Could you check a few things on this drawing? It's one solid part, dimensions in mm from its lowest x, y, z. A direction names the side the tool comes from. Give positions to 0.01 mm unless a question says otherwise; leave off trailing zeros. Write each loop counter-clockwise with the first axis right and the second up, starting at its lowest first coordinate (ties: lowest second). Pieces come first, ordered by that corner, then holes. Notation, with made-up numbers: (31.5, 23) - (69.5, 23) arc R14 cw to (69.5, 29) - close; hole circle Ø9 at (29.25, -17). An arc over 180 degrees is marked (long way). One line per item, written item: value. Start each with the question number.
1) On a 3-axis mill with a long thin cutter (end or side, diameter ignored), from which of +Z, -Z, +X, -X, +Y, -Y can I reach the whole of each face in a straight line? I mean the marked faces 1, 2 and 3. Say none if no direction works.
2) Imagine slicing it at B-B on x = 4. Write out the boundary of the cut face in (y, z).
3) Imagine slicing it at C-C on y = 8. Write out the boundary of the cut face in (x, z), plus the area to 3 significant figures.
4) Imagine slicing it at A-A on z = 4. Write out the boundary of the cut face in (x, y).
5) Please list where these lines run through material, in increasing order: L1, parallel to Y at x = 6.5, z = 3.75; L2, parallel to X at y = 7, z = 4; L3, parallel to X at y = 44.5, z = 1.5. Write a range as [from, to].
6) Imagine slicing it at D-D on y = 25.5. Write out the boundary of the cut face in (x, z).
7) I'm going to push a flat-ended pin straight in: P1, Ø1.5, axis at y = 11.5, z = 6.5, coming from the +X side. Where does the tip first touch, or does it pass through?
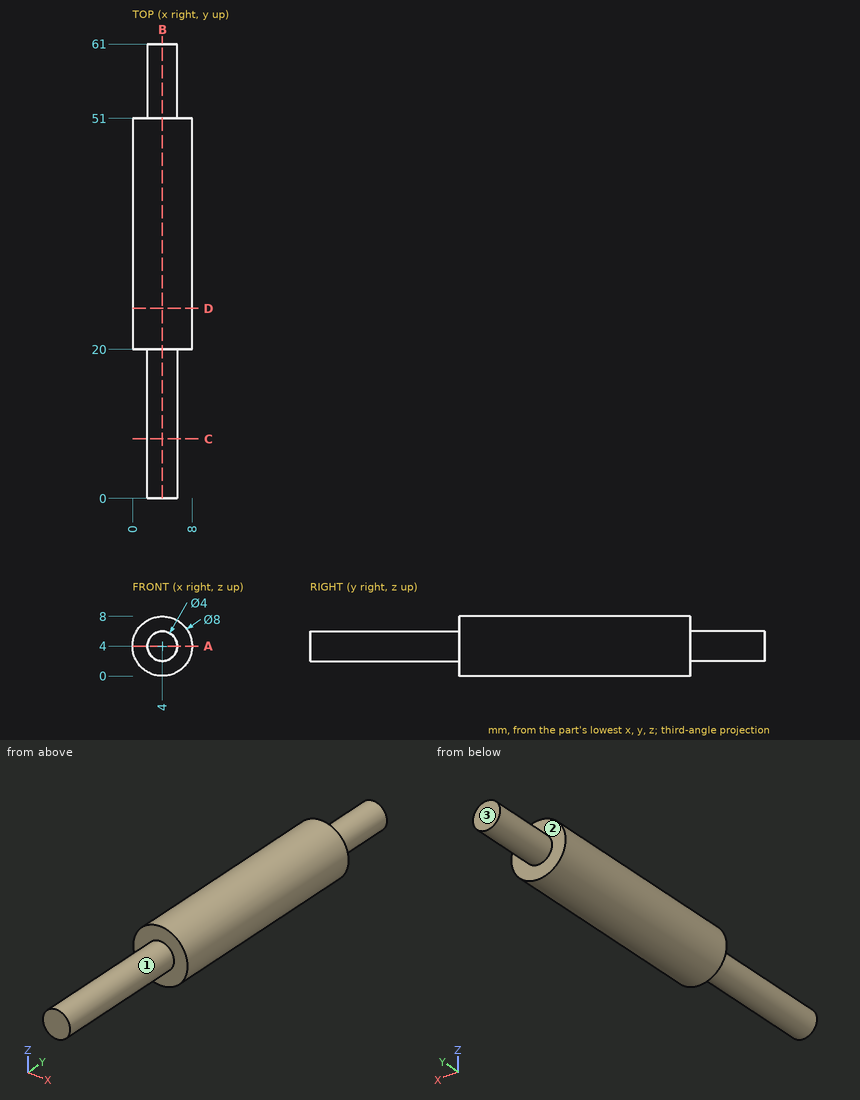
Numbers:
1. face 1: -Y
1. face 2: +Y
1. face 3: +Z, -Z, +X, -X, +Y
2. outline: (0, 2) - (20, 2) - (20, 0) - (51, 0) - (51, 2) - (61, 2) - (61, 6) - (51, 6) - (51, 8) - (20, 8) - (20, 6) - (0, 6) - close
3. outline: circle Ø4 at (4, 4)
3. area: 12.6 mm^2
4. outline: (0, 20) - (2, 20) - (2, 0) - (6, 0) - (6, 20) - (8, 20) - (8, 51) - (6, 51) - (6, 61) - (2, 61) - (2, 51) - (0, 51) - close
5. L1: [20, 51]
5. L2: [2, 6]
5. L3: [0.88, 7.12]
6. outline: circle Ø8 at (4, 4)
7. P1: x = 4.97
